```python
from build123d import *

# Parameters (mm, degrees)
F0_R     = 124
F1_DEPTH = 260
F2_R     = 124
F3_DEPTH = 34
F4_R     = 124
F5_DEPTH = 34
F6_R     = 10
F7_DEPTH = 16


with BuildPart() as f1:
    # F0 (on Front) → F1 (new body)
    with BuildSketch(Plane.XZ):
        Polygon((490, 0), (30, 0), (30, -36), (0, -36), (0, -248), (30, -248), (30, -284), (490, -284), (490, -248), (520, -248), (520, -36), (490, -36), align=None)
        with Locations((260, -142)):
            Circle(F0_R, mode=Mode.SUBTRACT)
    extrude(amount=F1_DEPTH)

    # F2 (on face) → F3 (cut)
    with BuildSketch(Plane.XZ.offset(260)):
        with BuildLine():
            Line((149.3835455278, -284), (370.6164544722, -284))
            ThreePointArc((370.6164544722, -284), (440, -142), (370.6164544722, 0))
            Line((370.6164544722, 0), (149.3835455278, 0))
            ThreePointArc((149.3835455278, 0), (80, -142), (149.3835455278, -284))
        make_face()
        with Locations((260, -142)):
            Circle(F2_R, mode=Mode.SUBTRACT)
    extrude(amount=-F3_DEPTH, mode=Mode.SUBTRACT)

    # F4 (on face) → F5 (join)
    with BuildSketch(Plane(origin=(0, 0, 0), x_dir=(-1, 0, 0), z_dir=(0, 1, 0))):
        Polygon((-30, -36), (-30, 0), (-490, 0), (-490, -36), (-520, -36), (-520, -248), (-490, -248), (-490, -284), (-30, -284), (-30, -248), (0, -248), (0, -36), align=None)
        with Locations((-260, -142)):
            Circle(F4_R, mode=Mode.SUBTRACT)
        with Locations((-260, -142)):
            Circle(F4_R)
    extrude(amount=-F5_DEPTH)

    # F6 (on face) → F7 (cut)
    with BuildSketch(Plane.XZ.offset(226)):
        with Locations((170.6566416515, -19.029416855)):
            Circle(F6_R)
        with Locations((115.4394095231, -95.029416855)):
            Circle(F6_R)
        with Locations((115.4394095231, -188.970583145)):
            Circle(F6_R)
        with Locations((170.6566416515, -264.970583145)):
            Circle(F6_R)
        with Locations((349.3433583485, -264.970583145)):
            Circle(F6_R)
        with Locations((404.5605904769, -188.970583145)):
            Circle(F6_R)
        with Locations((404.5605904769, -95.029416855)):
            Circle(F6_R)
        with Locations((349.3433583485, -19.029416855)):
            Circle(F6_R)
    extrude(amount=-F7_DEPTH, mode=Mode.SUBTRACT)


solid = f1.part
```
Work out the finished part from the listing and answer in its coordinate system (mm). A direction names the side the tool comes from. Give positions to 0.01 mm unless a question says otherwise; leave off trailing zeros. Loops run counter-clockwise (first coordinate to the right, second up) from the corner with the lowest first, then second, coordinate; pieces in that order, holes last. Notation, with made-up numbers: (62, -22.75) - (94, -22.75) arc R11 cw to (94, -8.75) - close; hole circle Ø6 at (-2, 36). An arc over 180 degrees is marked (long way). One line per question, with ' | ' between items.
(1) The part is cut by section A-A (y = -135). Write down the section's boundary in (x, z), then the cut area to 3 significant figures.
Recorded:
outline: (0, -248) - (30, -248) - (30, -284) - (490, -284) - (490, -248) - (520, -248) - (520, -36) - (490, -36) - (490, 0) - (30, 0) - (30, -36) - (0, -36) - close; hole circle Ø248 at (260, -142) | area: 95,100 mm²
(2) The mould has two halves that part along Z. Classify faces 4 (the face through (80.015, -243.238, -139.709)), 5 (the face through (263, -128, 0)), 6 (the face through (256, 0, -140)): +Z half, -Z half, draft (parallel to the pull), parting line (faces both ways), or undercut.
Recorded:
face 4: undercut | face 5: +Z half | face 6: draft
(3) Straight lines are drawn through the part: probe 1 along X at (y, z) = (-123.5, -142); probe 2 along Z at (x, y) = (258.5, -195.5); probe 3 along X at (y, z) = (-111.5, -17.5). For each, find the intervals that lie inside material, in ascending order.
Recorded:
probe 1: x = 0 to 136, 384 to 520 | probe 2: z = -284 to -265.99, -18.01 to 0 | probe 3: x = 30 to 490
(4) The part is cut by section B-B (z = -142). Write down the section's boundary in (x, y).
Recorded:
outline: (0, -260) - (80, -260) - (80, -226) - (136, -226) - (136, -34) - (384, -34) - (384, -226) - (440, -226) - (440, -260) - (520, -260) - (520, 0) - (0, 0) - close
(5) The part is cut by section C-C (x = 260). Write down the section's boundary in (y, z), then the cut area to 3 significant figures.
Recorded:
outline: (-226, -284) - (0, -284) - (0, 0) - (-226, 0) - (-226, -18) - (-34, -18) - (-34, -266) - (-226, -266) - close | area: 16,600 mm²
(6) A tool of negligible diameter and unlimited length cuts with its end or side. For faces 1 (the face through (30, -128, -266)), 2 (the face through (490, -128, -18)), 3 (the face through (108.07, -218.11, -182.21)), from which of +Z, -Z, +X, -X, +Y, -Y can it reach the whole face along a straight path? Write none if from no direction.
Recorded:
face 1: -Z, -X, +Y, -Y | face 2: +Z, +X, +Y, -Y | face 3: -Y
(7) Each of these flat-tipped pins is pushed along its axis until it touches: pin 1 Ø22 at (x, z) = (402.5, -100) entering from -Y; pin 2 Ø6 at (x, z) = (349, -23.5) entering from -Y; pin 3 Ø5 at (x, z) = (212, -156.5) entering from -Y. Where does it stop, or does it pass through?
Recorded:
pin 1: stops at y = -226 | pin 2: stops at y = -210 | pin 3: stops at y = -34
(8) The part is cut by section D-D (z = -76). Write down the section's boundary in (x, y), then the cut area to 3 significant figures.
Recorded:
outline: (0, -260) - (92.54, -260) - (92.54, -226) - (155.02, -226) - (155.02, -34) - (364.98, -34) - (364.98, -226) - (427.46, -226) - (427.46, -260) - (520, -260) - (520, 0) - (0, 0) - close | area: 83,500 mm²
